Can you work these out from the drawing? Everything is in mm from the part's minimum corner. Round coordinates to 2 decimals unless told otherwise and drop trailing zeros. Loops run counter-clockwise (first coordinate to the right, second up) from the corner with the lowest first, then second, coordinate; pieces in that order, holes last. Notation, with made-up numbers: (4.25, 55.25) -> (25.25, 55.25) arc R21 cw to (25.25, 78.25) -> close; hole circle Ø7 at (10.5, 82). An arc over 180 degrees is marked (long way). One line per item, written item: value.
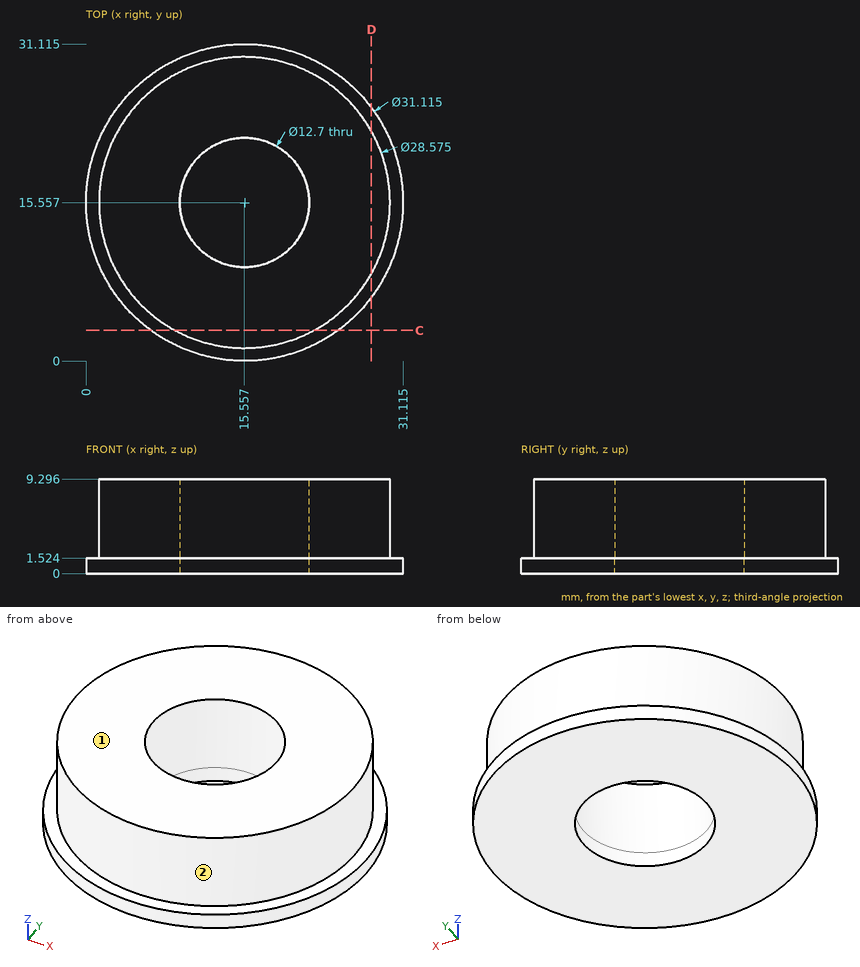
Item 1: If we section it at D-D on x = 28: List the corners of the cut face in (y, z) for me (1 decimal).
Output:
outline: (6.2, 0) -> (24.9, 0) -> (24.9, 1.5) -> (22.6, 1.5) -> (22.6, 9.3) -> (8.5, 9.3) -> (8.5, 1.5) -> (6.2, 1.5) -> close
Item 2: If we mould it in two halves opening along Y, with no side actions, what happens to the marked faces 1 and 2? For each: released by +Y, released by -Y, zero draft, split by the parting line, or undercut.
Output:
face 1: zero draft
face 2: split by the parting line
Item 3: If we section it at C-C on y = 3: List the corners of the cut face in (x, z) for me (1 decimal).
Output:
outline: (6.4, 0) -> (24.7, 0) -> (24.7, 1.5) -> (22.4, 1.5) -> (22.4, 9.3) -> (8.7, 9.3) -> (8.7, 1.5) -> (6.4, 1.5) -> close
Item 4: I need wall thicknesses on line 1 (X direction, y = 19.5, z = 4) (1 decimal); line 2 (Y direction, x = 15.5, z = 7.75) (1 decimal); line 3 (Y direction, x = 19, z = 2) (1 decimal). Which ranges of each line are inside material? Lowest first, please. Write a range as from..to.
Output:
line 1: x = 1.8..10.6, 20.5..29.3
line 2: y = 1.3..9.2, 21.9..29.8
line 3: y = 1.7..10.2, 20.9..29.4
Item 5: Will these pins go through, and if not, where does the flat tip stop? pin 1 Ø1.5 at (x, z) = (4.5, 7.5) entering from -Y (1 decimal); pin 2 Ø2 at (x, z) = (11, 5) entering from -Y; pin 3 Ø2 at (x, z) = (15, 3) entering from +Y (1 decimal); pin 4 Ø1.5 at (x, y) = (12, 12.5) entering from +Z.
Output:
pin 1: stops at y = 5.7
pin 2: stops at y = 1.72
pin 3: stops at y = 29.8
pin 4: passes through
